Autodesk Inventor part; units mm, degrees
ref_plane "YZ Plane" through (0, 0, 0) normal (1, 0, 0) x (0, 1, 0)
ref_plane "XZ Plane" through (0, 0, 0) normal (0, 1, 0) x (-1, 0, 0)
ref_plane "XY Plane" through (0, 0, 0) normal (0, 0, 1) x (1, 0, 0)
sketch "Sketch1" plane through (0, 0, 0) normal (0, 0, 1) x (1, 0, 0)
  circle A0 centre (0, -0.002) radius 1.375
  circle A1 centre (-0.0001, 26.2) radius 1.5
  line L0 (0, -0.002) -> (0, -4.002)
  line L1 (0, -4.002) -> (-3, -4.002)
  line L2 (-0.0001, 26.2) -> (-3, 26.2)
  line L3 (-3, 26.2) -> (-3, 30.2)
  line L4 (-3, 30.2) -> (3, 30.2)
  line L5 (-3, -4.002) -> (3, -4.002)
  line L6 (3, -4.002) -> (3, 30.2)
  line L7 (3, 30.2) -> (-3, 30.2)
  line L8 (-3, 30.2) -> (-3, -4.002)
  circle A2 centre (0, -0.002) radius 1.625
  circle A3 centre (42.1135, 26.2) radius 1.5
  circle A4 centre (-0.0001, 26.2) radius 1.5
  line L9 (-6.8272, 34.4) -> (15.5728, 34.4)
  line L10 (-6.8272, 17) -> (-6.8272, 34.4)
  line L11 (48.6728, 17) -> (-6.8272, 17)
  line L12 (48.6728, 34.4) -> (48.6728, 17)
  line L13 (26.2804, 34.4) -> (48.6728, 34.4)
  line L14 (26.2804, 47.56) -> (26.2804, 34.4)
  line L15 (15.5728, 47.56) -> (26.2804, 47.56)
  line L16 (15.5728, 34.4) -> (15.5728, 47.56)
  circle A5 centre (20.9266, 44.75) radius 1.75
  circle A6 centre (-0.0001, 26.2) radius 1.625
  point P0 (0, 0)
  dimension "d0" = 4
  dimension "d1" = 3
  dimension "d2" = 4
  dimension "d3" = 6
  dimension "d4" = 3.25
  dimension "d5" = 3.25
extrude "Extrusion1" add sketch "Sketch1" along normal blind 2 contours L1 L8 L11 L6 L5 | L8 L3 L4 L6 L11
fillet "Fillet1" radius 1 4 edges at (-3, -4.002, 1) (3, -4.002, 1) (3, 30.2, 1) (-3, 30.2, 1)
properties part number "SyringeBarTail"
Source: CAD feature listing. Evaluate the final solid. Frame: model axes, mm. Round coordinates to 2 decimals unless told otherwise and drop trailing zeros. Loops run counter-clockwise (first coordinate to the right, second up) from the corner with the lowest first, then second, coordinate; pieces in that order, holes last. Notation, with made-up numbers: M -28,4 L -9,4 A6 cw -9,12 Z; hole C -36,1.25 d1. An arc over 180 degrees is marked long. Return JSON: item names as keys, results as strings. Group by question number.
1. Section query B-B on x = 0. Output: boundary loops of the cut face in (y, z) (3 decimals).
2. Pin query (flat end, axial travel): pin 1 (3 mm diameter, centred on x = 0, y = 26.2, fed in from +Z). Return the tip coordinate at first contact, or that it passes through.
3. Material intervals for line 1 along Y through (x, z) = (0, 0.95) (3 decimals); line 2 along X through (y, z) = (26.2, 1.55); line 3 along Y through (x, z) = (-0.55, 1.9), sorted ascending. Write a range as from..to.
4. Section query D-D on y = -1. Output: boundary loops of the cut face in (x, z), and give its area (3 significant figures).
5. Mould query, pull axis Y, two halves, no side actions, for faces 1 (the face through (2.715, 29.899, 1.014)), 2 (the face through (-3, 13, 1)), 3 (the face through (-1.29, 0.987, 0.986)). Classes: released by +Y, released by -Y, zero draft, split by the parting line, or undercut.
6. Section query A-A on y = 26.2. Output: boundary loops of the cut face in (x, z), and give its area (3 significant figures).
7. Section query C-C on z = 1.25. Output: boundary loops of the cut face in (x, y) (3 decimals), and give its area (3 significant figures).
Checks:
{
 "1": {"outline": "M -4.002,0 L -1.627,0 L -1.627,2 L -4.002,2 Z; M 1.623,0 L 24.575,0 L 24.575,2 L 1.623,2 Z; M 27.825,0 L 30.2,0 L 30.2,2 L 27.825,2 Z"},
 "2": {"pin 1": "passes through"},
 "3": {"line 1": "y = -4.002..-1.627, 1.623..24.575, 27.825..30.2", "line 2": "x = -3..-1.63, 1.62..3", "line 3": "y = -4..-1.53, 1.53..24.67, 27.73..30.2"},
 "4": {"outline": "M -3,0 L -1.28,0 L -1.28,2 L -3,2 Z; M 1.28,0 L 3,0 L 3,2 L 1.28,2 Z", "area": "6.87 mm²"},
 "5": {"face 1": "released by +Y", "face 2": "zero draft", "face 3": "undercut"},
 "6": {"outline": "M -3,0 L -1.63,0 L -1.63,2 L -3,2 Z; M 1.62,0 L 3,0 L 3,2 L 1.62,2 Z", "area": "5.50 mm²"},
 "7": {"outline": "M -3,-3.002 A1 ccw -2,-4.002 L 2,-4.002 A1 ccw 3,-3.002 L 3,29.2 A1 ccw 2,30.2 L -2,30.2 A1 ccw -3,29.2 Z; hole C 0,-0.002 d3.25; hole C 0,26.2 d3.25", "area": "188 mm²"}
}
